```python
from build123d import *

# Parameters (mm, degrees)
SKETCH1_R           = 10
BOSS_EXTRUDE1_DEPTH = 10
HOLE2_D             = 7
HOLE2_CBORE_D       = 10
HOLE2_CBORE_DEPTH   = 5


with BuildPart() as part:
    # Sketch1 → Boss-Extrude1 (new body)
    with BuildSketch(Plane.XY):
        with BuildLine():
            Line((600, -600), (600, 600))
            ThreePointArc((600, 600), (0, 1200), (-600, 600))
            Line((-600, 600), (-600, -600))
            ThreePointArc((-600, -600), (0, -1200), (600, -600))
        make_face()
        with Locations((0, 1150)):
            Circle(SKETCH1_R, mode=Mode.SUBTRACT)
        with Locations((-550, 600)):
            Circle(SKETCH1_R, mode=Mode.SUBTRACT)
        with Locations((-550, 0)):
            Circle(SKETCH1_R, mode=Mode.SUBTRACT)
        with Locations((-550, -600)):
            Circle(SKETCH1_R, mode=Mode.SUBTRACT)
        with Locations((550, 600)):
            Circle(SKETCH1_R, mode=Mode.SUBTRACT)
        with Locations((550, 0)):
            Circle(SKETCH1_R, mode=Mode.SUBTRACT)
        with Locations((550, -600)):
            Circle(SKETCH1_R, mode=Mode.SUBTRACT)
        with Locations((0, -1150)):
            Circle(SKETCH1_R, mode=Mode.SUBTRACT)
        with BuildLine():
            Line((450, -600), (450, 600))
            ThreePointArc((450, 600), (0, 1050), (-450, 600))
            Line((-450, 600), (-450, -600))
            ThreePointArc((-450, -600), (0, -1050), (450, -600))
        make_face(mode=Mode.SUBTRACT)
    extrude(amount=-BOSS_EXTRUDE1_DEPTH)

    # Hole2 (through all)
    with Locations(Plane(origin=(475, 19.25, -10), x_dir=(-1, 0, 0), z_dir=(0, 0, -1))):
        with Locations((0, 0), (0, 480), (0, -480)):
            hole2 = CounterBoreHole(HOLE2_D / 2, HOLE2_CBORE_D / 2, HOLE2_CBORE_DEPTH)

    # Mirror1: Hole2 across plane
    add(hole2.mirror(Plane(origin=(0, 0, 0), x_dir=(0, 0, 1), z_dir=(1, 0, 0))), mode=Mode.SUBTRACT)


solid = part.part
```
Can you work these out from the model? Positions are in its coordinate system, mm. A direction names the side the tool comes from. Coordinates: 2 decimals unless noted, no trailing zeros. Loops run counter-clockwise (first coordinate to the right, second up) from the corner with the lowest first, then second, coordinate; pieces in that order, holes last.
Item 1: Suppose I cut it at C-C (x = 516.5). Please give me the cut outline in (y, z), then the cut area to 3 significant figures.
Answers below:
outline: (-905.33, -10) - (905.33, -10) - (905.33, 0) - (-905.33, 0) - close
area: 18,100 mm2
Item 2: I'm going to push flat-ended pins straight in: pin 1 (1 mm diameter, centred on x = -253, z = -2.5, fed in from +Y); pin 2 (12 mm diameter, centred on x = 0, y = 1150, fed in from -Z); pin 3 (3 mm diameter, centred on x = -477, y = 21, fed in from -Z); pin 4 (1 mm diameter, centred on y = 839, z = -2.5, fed in from +X). Where does each tip first touch, or does it pass through?
Answers below:
pin 1: stops at y = 1144.28
pin 2: passes through
pin 3: stops at z = -5
pin 4: stops at x = 550.56
Item 3: If we mould it in two halves opening along Y, with no side actions, what happens to faces 3 (the face through (13.194, 1199.855, -4.93)), 4 (the face through (-492, 6, -10)), 5 (the face through (9.9, 1049.89, -4.93))? For each: released by +Y, released by -Y, zero draft, split by the parting line, or undercut.
Answers below:
face 3: released by +Y
face 4: zero draft
face 5: undercut
Item 4: Suppose I cut it at A-A (y = -201). Please give me the cut outline in (x, z), then the cut area to 3 significant figures.
Answers below:
outline: (-600, -10) - (-450, -10) - (-450, 0) - (-600, 0) - close; (450, -10) - (600, -10) - (600, 0) - (450, 0) - close
area: 3,000 mm2
Item 5: Please list where these lines run through material, in increasing order: L1, parallel to X at y = 600, z = -8; L2, parallel to X at y = -460.75, z = -6.7; L3, parallel to X at y = 380.5, z = -5.75.
Answers below:
L1: x = -600 to -560, -540 to -450, 450 to 540, 560 to 600
L2: x = -600 to -480, -470 to -450, 450 to 470, 480 to 600
L3: x = -600 to -450, 450 to 600
Item 6: Which directions (+Z, -Z, +X, -X, +Y, -Y) give clear straight access to the entire face, cutting with the end or side of a thin tool? Please do faces 1 (the face through (-13.194, -1199.855, -4.93)), 2 (the face through (-9.9, -1049.89, -4.93)).
Answers below:
face 1: +Z, -Z, -Y
face 2: +Z, -Z
Item 7: Suppose I cut it at B-B (x = -54.5). Please give me the cut outline in (y, z).
Answers below:
outline: (-1197.52, -10) - (-1046.69, -10) - (-1046.69, 0) - (-1197.52, 0) - close; (1046.69, -10) - (1197.52, -10) - (1197.52, 0) - (1046.69, 0) - close
